The model under review builds one solid part; all positions refer to its coordinate system, in mm. A direction names the side the tool comes from. Round coordinates to 2 decimals unless told otherwise and drop trailing zeros. Write each loop counter-clockwise with the first axis right and the second up, starting at its lowest first coordinate (ties: lowest second). Pieces come first, ordered by that corner, then holes. Notation, with made-up numbers: (26.25, -18.5) -> (35.25, -18.5) arc R24 cw to (35.25, 11.5) -> close; hole circle Ø7 at (-39, 60). An arc over 180 degrees is marked (long way). Use CSV: the item, a comma, the result in double quotes. Start each with the question number.
1) Take a section at C-C, the plane y = -7.25. State how many separate pieces and enclosed holes the cut face has, then the cut area to 3 significant figures.
2) Machinability: for faces 1 (the face through (23, -5, -18)), 2 (the face through (-72.5, -5, 7)), which of the approach directions +Z, -Z, +X, -X, +Y, -Y give a long, thin tool a straight path to every point of the face, cutting with its end or side? Answer none if there is none.
3) For pin 1 Ø5 at (x, y) = (42, -3) entering from +Z; pin 2 Ø2.5 at (y, z) = (-7, 57) entering from +X; pin 3 Ø4 at (y, z) = (-4.5, 54) entering from -X; pin 4 Ø1.5 at (x, z) = (15, 9.5) entering from +Y, all flat-tipped, find the tip position at first contact; note any pin that passes through.
4) Take a section at B-B, the plane x = 15.5. Give the boundary of the cut face in (y, z), then the cut area to 3 significant figures.
5) Mouldability with a two-part tool opening along Z and no side actions: class faces 3 (the face through (-61.094, -5.07, 61.972)), 4 (the face through (72.5, -5, 7)), 5 (the face through (-23, -4.9, -34.4)) as released by +Z, released by -Z, zero draft, split by the parting line, or undercut.
6) Wall thickness on probe 1 along X at (y, z) = (-0.25, -2.5); probe 2 along Z at (x, y) = (0, -3.5); probe 3 along X at (y, z) = (-7.75, 28.5): over which ranges is each line inside the solid? List them lowest first. Write a range as [from, to].
7) Take a section at A-A, the plane z = -6.5. Give the boundary of the cut face in (x, y), then the cut area to 3 significant figures.
from build123d import *

# Parameters (mm, degrees)
SKETCH_W  = 145
SKETCH_H  = 133.4
SKETCH_R  = 10
PAD_DEPTH = 10
FILLET_R  = 40


with BuildPart() as part:
    # Sketch → Pad (new body)
    with BuildSketch(Plane.XZ):
        with Locations((0, 7.3)):
            Rectangle(SKETCH_W, SKETCH_H)
        with Locations((0, 39.5)):
            Circle(SKETCH_R, mode=Mode.SUBTRACT)
        with BuildLine():
            ThreePointArc((-13.5, 59), (-15.5, 61), (-17.5, 59))
            Line((-17.5, 59), (-17.5, 51))
            ThreePointArc((-17.5, 51), (-15.5, 49), (-13.5, 51))
            Line((-13.5, 59), (-13.5, 51))
        make_face(mode=Mode.SUBTRACT)
        with BuildLine():
            ThreePointArc((17.5, 59), (15.5, 61), (13.5, 59))
            Line((13.5, 59), (13.5, 51))
            ThreePointArc((13.5, 51), (15.5, 49), (17.5, 51))
            Line((17.5, 59), (17.5, 51))
        make_face(mode=Mode.SUBTRACT)
        with BuildLine():
            ThreePointArc((-13.5, 28), (-15.5, 30), (-17.5, 28))
            Line((-17.5, 28), (-17.5, 20))
            ThreePointArc((-17.5, 20), (-15.5, 18), (-13.5, 20))
            Line((-13.5, 28), (-13.5, 20))
        make_face(mode=Mode.SUBTRACT)
        with BuildLine():
            ThreePointArc((17.5, 28), (15.5, 30), (13.5, 28))
            Line((13.5, 28), (13.5, 20))
            ThreePointArc((13.5, 20), (15.5, 18), (17.5, 20))
            Line((17.5, 28), (17.5, 20))
        make_face(mode=Mode.SUBTRACT)
        with BuildLine():
            ThreePointArc((-21, -20), (-23, -18), (-25, -20))
            Line((-25, -20), (-25, -28))
            ThreePointArc((-25, -28), (-23, -30), (-21, -28))
            Line((-21, -20), (-21, -28))
        make_face(mode=Mode.SUBTRACT)
        with BuildLine():
            ThreePointArc((25, -20), (23, -18), (21, -20))
            Line((21, -20), (21, -28))
            ThreePointArc((21, -28), (23, -30), (25, -28))
            Line((25, -20), (25, -28))
        make_face(mode=Mode.SUBTRACT)
        with BuildLine():
            ThreePointArc((-21, -36.4), (-23, -34.4), (-25, -36.4))
            Line((-25, -36.4), (-25, -44.4))
            ThreePointArc((-25, -44.4), (-23, -46.4), (-21, -44.4))
            Line((-21, -36.4), (-21, -44.4))
        make_face(mode=Mode.SUBTRACT)
        with BuildLine():
            ThreePointArc((25, -36.4), (23, -34.4), (21, -36.4))
            Line((21, -36.4), (21, -44.4))
            ThreePointArc((21, -44.4), (23, -46.4), (25, -44.4))
            Line((25, -36.4), (25, -44.4))
        make_face(mode=Mode.SUBTRACT)
        with BuildLine():
            ThreePointArc((-54.5, 20), (-57.5, 23), (-60.5, 20))
            Line((-60.5, 20), (-60.5, -20))
            ThreePointArc((-60.5, -20), (-57.5, -23), (-54.5, -20))
            Line((-54.5, 20), (-54.5, -20))
        make_face(mode=Mode.SUBTRACT)
        with BuildLine():
            ThreePointArc((60.5, 20), (57.5, 23), (54.5, 20))
            Line((54.5, 20), (54.5, -20))
            ThreePointArc((54.5, -20), (57.5, -23), (60.5, -20))
            Line((60.5, 20), (60.5, -20))
        make_face(mode=Mode.SUBTRACT)
    extrude(amount=PAD_DEPTH)

    # Fillet
    fillet_edges = [part.edges().sort_by_distance(p)[0] for p in [
        (-72.5, -5, 74),
        (72.5, -5, 74),
        (72.5, -5, -59.4),
        (-72.5, -5, -59.4),
    ]]
    fillet(fillet_edges, radius=FILLET_R)


solid = part.part
Values found:
1,separate pieces,"1"
1,enclosed holes,"11"
1,area,"16,800 mm²"
2,face 1,"+Y, -Y"
2,face 2,"+Z, -Z, -X, +Y, -Y"
3,pin 1,"z = 73.38"
3,pin 2,"x = 66.07"
3,pin 3,"x = -68.22"
3,pin 4,"y = 0"
4,outline,"(-10, -59.4) -> (0, -59.4) -> (0, 18) -> (-10, 18) -> close; (-10, 30) -> (0, 30) -> (0, 49) -> (-10, 49) -> close; (-10, 61) -> (0, 61) -> (0, 74) -> (-10, 74) -> close"
4,area,"1,090 mm²"
5,face 3,"released by +Z"
5,face 4,"zero draft"
5,face 5,"undercut"
6,probe 1,"[-72.5, -60.5], [-54.5, 54.5], [60.5, 72.5]"
6,probe 2,"[-59.4, 29.5], [49.5, 74]"
6,probe 3,"[-72.5, -17.44], [-13.56, 13.56], [17.44, 72.5]"
7,outline,"(-72.5, -10) -> (-60.5, -10) -> (-60.5, 0) -> (-72.5, 0) -> close; (-54.5, -10) -> (54.5, -10) -> (54.5, 0) -> (-54.5, 0) -> close; (60.5, -10) -> (72.5, -10) -> (72.5, 0) -> (60.5, 0) -> close"
7,area,"1,330 mm²"
